The drawing under review shows one solid part. Ordinate dimensions are in mm from its lowest x, y, z. Give positions to 0.01 mm unless a question says otherwise; leave off trailing zeros. Order: outer loops, then holes, each group sorted by start corner. A loop starts at its lowest first (then second) coordinate and runs counter-clockwise, first axis right, second up. Notation, with made-up numbers: (68, 9) - (123, 9) arc R26 cw to (123, 34) - close; hole circle Ø9 at (45.25, 47.5). An arc over 180 degrees is marked (long way). Use CSV: the item, a comma, the result in double quotes.
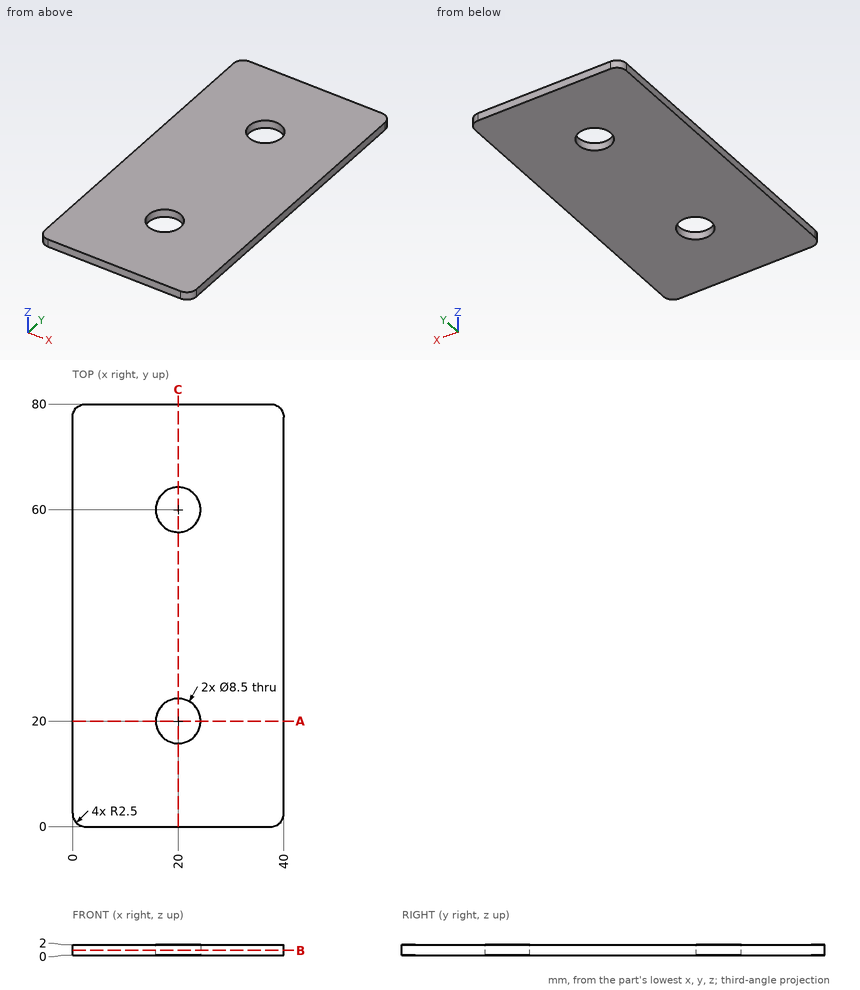
Item 1: Wall thickness on L1, parallel to Y at x = 20, z = 1.4; L2, parallel to X at y = 23.5, z = 1.5: over which ranges is each line inside the solid? List them lowest first.
Results list:
L1,"y = 0 to 15.75, 24.25 to 55.75, 64.25 to 80"
L2,"x = 0 to 17.59, 22.41 to 40"
Item 2: Take a section at A-A, the plane y = 20. Give the boundary of the cut face in (x, z), and give its area (3 significant figures).
Results list:
outline,"(0, 0) - (15.75, 0) - (15.75, 2) - (0, 2) - close; (24.25, 0) - (40, 0) - (40, 2) - (24.25, 2) - close"
area,"63.0 mm2"
Item 3: Take a section at B-B, the plane z = 0.9. Give the boundary of the cut face in (x, y).
Results list:
outline,"(0, 2.5) arc R2.5 ccw to (2.5, 0) - (37.5, 0) arc R2.5 ccw to (40, 2.5) - (40, 77.5) arc R2.5 ccw to (37.5, 80) - (2.5, 80) arc R2.5 ccw to (0, 77.5) - close; hole circle Ø8.5 at (20, 20); hole circle Ø8.5 at (20, 60)"
Item 4: Take a section at C-C, the plane x = 20. Give the boundary of the cut face in (y, z).
Results list:
outline,"(0, 0) - (15.75, 0) - (15.75, 2) - (0, 2) - close; (24.25, 0) - (55.75, 0) - (55.75, 2) - (24.25, 2) - close; (64.25, 0) - (80, 0) - (80, 2) - (64.25, 2) - close"
